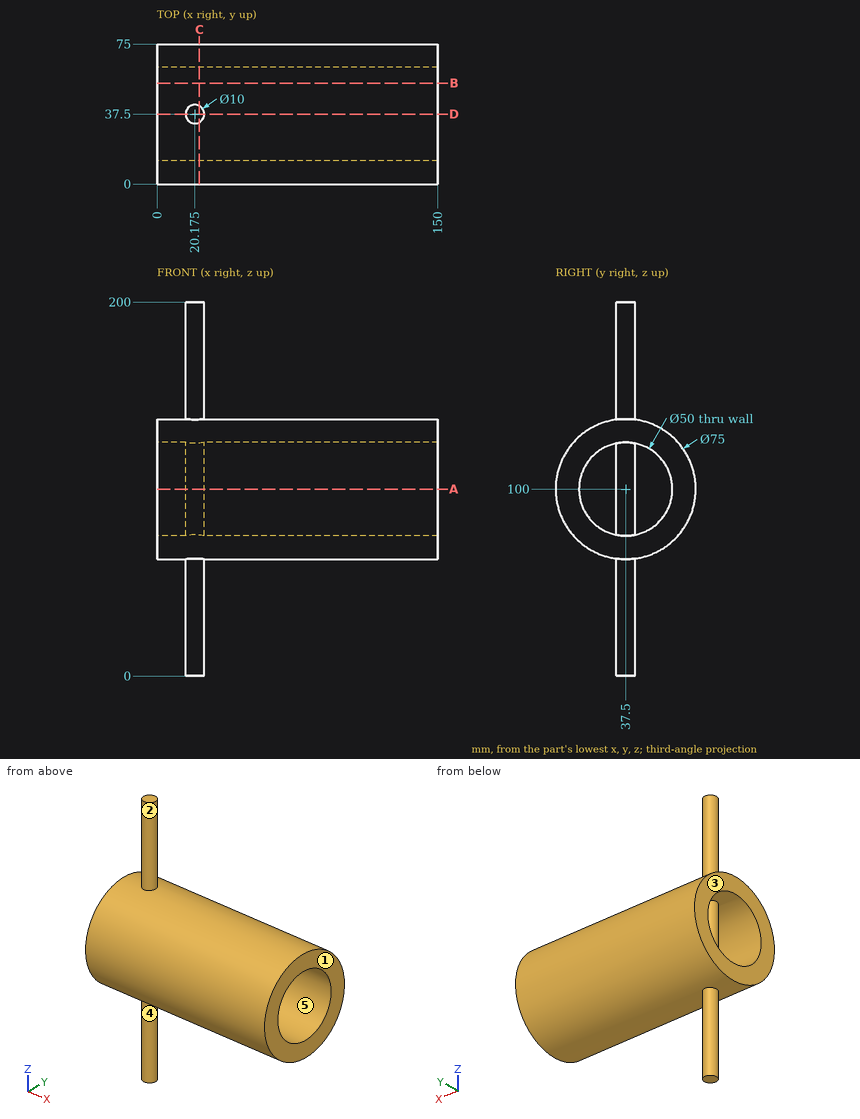
Geometry: see drawing. Coordinates: mm, zero at the bounding-box minimum. A direction names the side the tool comes from. Give positions to 0.01 mm unless a question says otherwise; leave off trailing zeros. Write each loop counter-clockwise with the first axis right and the second up, starting at its lowest first coordinate (ties: lowest second). Pieces come first, ordered by that corner, then holes. Notation, with made-up numbers: (-11, 74.5) -> (19, 74.5) arc R31 cw to (19, 103.5) -> close; hole circle Ø4 at (76, 7). An arc over 180 degrees is marked (long way). Use one line per item in the form item = value. Start each with the question number.
1) Section query D-D on y = 37.5. Return the cut outline in (x, z) (1 decimal).
2) Section query A-A on z = 100. Return the cut outline in (x, y) (1 decimal), then the cut area to 3 significant figures.
3) Pin query (flat end, axial travel): pin 1 (3 mm diameter, centred on x = 28.5, y = 49.5, fed in from -Z); pin 2 (12 mm diameter, centred on y = 45, z = 45.5, fed in from +X) (1 decimal); pin 3 (2 mm diameter, centred on x = 16.5, z = 73.5, fed in from -Y) (1 decimal). Return the tip coordinate at first contact, or that it passes through.
4) Section query B-B on y = 54. Return the cut outline in (x, z) (1 decimal).
5) Ray query, probe 1 along Y at (x, z) = (53, 100); probe 2 along Z at (x, y) = (74, 37) (1 decimal); probe 3 along Y at (x, z) = (36.5, 119.5) (1 decimal). Return the intervals inside material, ascending. Write a range as from..to.
6) Section query C-C on x = 22.5. Return the cut outline in (y, z) (1 decimal), then the cut area to 3 significant figures.
7) Draft query along Y for the marked faces 3, 4 and 5. Return one class per face: pulls with the +Y half, pulls with the -Y half, needs draft (parallel to the pull), parting line crosses it, or undercut.
8) Set-up query: the marked faces 1 and 2. Return all of +Z, -Z, +X, -X, +Y, -Y with unobstructed straight access to the full face (end or side cutting, diameter ignored); none if empty.
Outcome:
q1.outline = (0, 62.5) -> (15.2, 62.5) -> (15.2, 0) -> (25.2, 0) -> (25.2, 62.5) -> (150, 62.5) -> (150, 75) -> (25.2, 75) -> (25.2, 125) -> (150, 125) -> (150, 137.5) -> (25.2, 137.5) -> (25.2, 200) -> (15.2, 200) -> (15.2, 137.5) -> (0, 137.5) -> (0, 125) -> (15.2, 125) -> (15.2, 75) -> (0, 75) -> close
q2.outline = (0, 0) -> (150, 0) -> (150, 12.5) -> (0, 12.5) -> close; (0, 62.5) -> (150, 62.5) -> (150, 75) -> (0, 75) -> close; circle Ø10 at (20.2, 37.5)
q2.area = 3,830 mm^2
q3.pin_1 = 64
q3.pin_2 = 24.9
q3.pin_3 = 10
q4.outline = (0, 66.3) -> (150, 66.3) -> (150, 81.2) -> (0, 81.2) -> close; (0, 118.8) -> (150, 118.8) -> (150, 133.7) -> (0, 133.7) -> close
q5.probe_1 = 0..12.5, 62.5..75
q5.probe_2 = 62.5..75, 125..137.5
q5.probe_3 = 5.5..21.9, 53.1..69.5
q6.outline = (33.1, 0) -> (41.9, 0) -> (41.9, 62.8) arc R37.5 ccw to (41.9, 137.2) -> (41.9, 200) -> (33.1, 200) -> (33.1, 137.2) arc R37.5 ccw to (33.1, 62.8) -> close; hole (33.1, 75.4) -> (33.1, 124.6) arc R25 ccw to start; hole (41.9, 75.4) arc R25 ccw to (41.9, 124.6) -> close
q6.area = 4,000 mm^2
q7.face_3 = needs draft
q7.face_4 = parting line crosses it
q7.face_5 = undercut
q8.face_1 = +Z, -Z, +X, +Y, -Y
q8.face_2 = +Z
